Geometry: see drawing. Coordinates: mm, zero at the bounding-box minimum. Give positions to 0.01 mm unless a question says otherwise; leave off trailing zeros. Write each loop counter-clockwise with the first axis right and the second up, starting at its lowest first coordinate (ties: lowest second). Pieces come first, ordered by that corner, then holes. Notation, with made-up numbers: (13, -31) -> (19, -31) arc R28 cw to (19, -12) -> close; hole circle Ø6 at (-2, -30). An arc over 180 degrees is marked (long way). Write item = value, one per line.
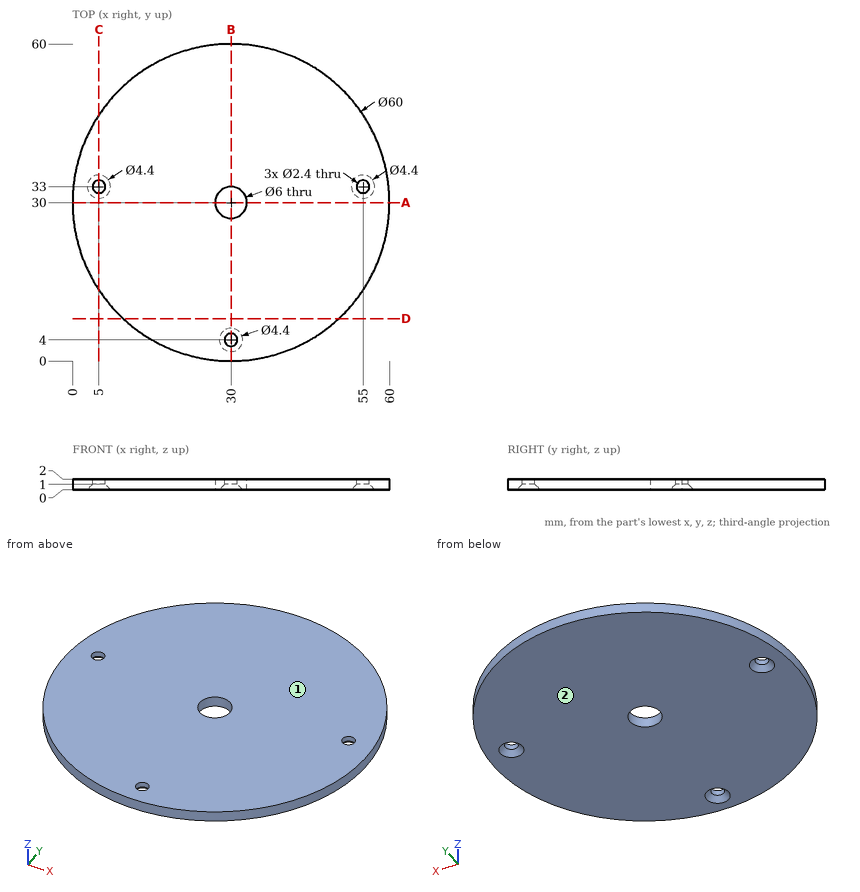
(1) Section query A-A (y = 30). Return loops of the section in (x, z).
Values follow:
outline = (0, 0) -> (27, 0) -> (27, 2) -> (0, 2) -> close; (33, 0) -> (60, 0) -> (60, 2) -> (33, 2) -> close
(2) Section query D-D (y = 8). Return loops of the section in (x, z), plus the area to 3 significant figures.
Values follow:
outline = (9.6, 0) -> (50.4, 0) -> (50.4, 2) -> (9.6, 2) -> close
area = 81.6 mm2
(3) Material intervals for line 1 (Y direction, x = 30, z = 1.65); line 2 (Y direction, x = 30, z = 0.75); line 3 (Y direction, x = 5, z = 1.6), sorted ascending.
Values follow:
line_1 = 0 to 2.8, 5.2 to 27, 33 to 60
line_2 = 0 to 2.55, 5.45 to 27, 33 to 60
line_3 = 13.42 to 31.8, 34.2 to 46.58
(4) Section query B-B (x = 30). Return loops of the section in (y, z).
Values follow:
outline = (0, 0) -> (1.8, 0) -> (2.8, 1) -> (2.8, 2) -> (0, 2) -> close; (5.2, 1) -> (6.2, 0) -> (27, 0) -> (27, 2) -> (5.2, 2) -> close; (33, 0) -> (60, 0) -> (60, 2) -> (33, 2) -> close
(5) Section query C-C (x = 5). Return loops of the section in (y, z).
Values follow:
outline = (13.42, 0) -> (30.8, 0) -> (31.8, 1) -> (31.8, 2) -> (13.42, 2) -> close; (34.2, 1) -> (35.2, 0) -> (46.58, 0) -> (46.58, 2) -> (34.2, 2) -> close
(6) Pull-direction query (Z, two-part tool) for the marked faces 1 and 2; classes: pulls with the +Z half, pulls with the -Z half, needs draft (parallel to the pull), parting line crosses it, or undercut.
Values follow:
face_1 = pulls with the +Z half
face_2 = pulls with the -Z half
